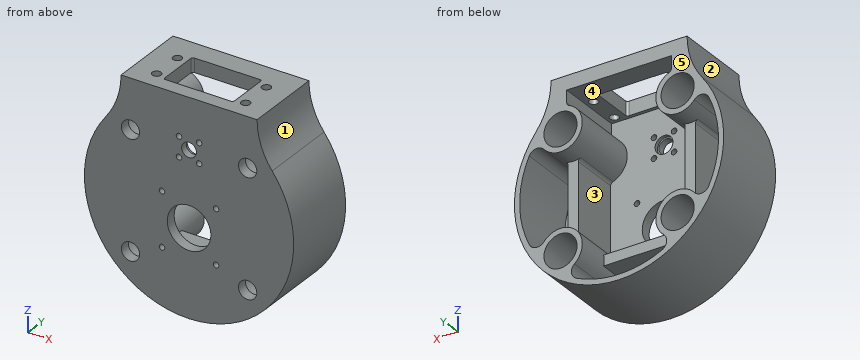
from build123d import *

# Parameters (mm, degrees)
SKETCH1_R           = 9.5
BOSS_EXTRUDE1_DEPTH = 45
BOSS_EXTRUDE2_DEPTH = 6
SKETCH3_R           = 5.25
SKETCH3_R_2         = 4.25
SKETCH3_R_3         = 1.6
CUT_EXTRUDE1_DEPTH  = 95.683683917
FILLET1_R           = 5
SKETCH4_R           = 5.1
CUT_EXTRUDE2_DEPTH  = 2
SKETCH5_R           = 12.5
SKETCH5_R_2         = 1.6
CUT_EXTRUDE3_DEPTH  = 98.308787031
CUT_EXTRUDE4_REACH  = 145.21
SKETCH6_W           = 40
SKETCH6_H           = 25
CUT_EXTRUDE5_REACH  = 145.21
SKETCH7_R           = 2.55
BOSS_EXTRUDE3_DEPTH = 28
FILLET2_R           = 2
BOSS_EXTRUDE4_DEPTH = 20
FILLET3_R           = 1.2


with BuildPart() as part:
    # Sketch1 → Boss-Extrude1 (new body)
    # profile 1 of 3: a face of its own
    with BuildSketch(Plane(origin=(0, 0, 0), x_dir=(1, 0, 0), z_dir=(0, 1, 0))):
        with BuildLine():
            ThreePointArc((-47.647058368, -36.465844689), (-41.21916632, -48.520286728), (-39, -62))
            Line((-39, -62), (39, -62))
            ThreePointArc((39, -62), (41.21916632, -48.520286728), (47.647058368, -36.465844689))
            ThreePointArc((47.647058368, -36.465844689), (0, 60), (-47.647058368, -36.465844689))
        make_face()
        with Locations(Location((-33.587572106, -33.587572106, 0), (0, 0, 90))):
            Circle(SKETCH1_R, mode=Mode.SUBTRACT)
        with Locations(Location((33.587572106, -33.587572106, 0), (0, 0, 90))):
            Circle(SKETCH1_R, mode=Mode.SUBTRACT)
        with BuildLine():
            Line((30, -54), (-30, -54))
            Line((-30, -54), (-30, -48.466483264))
            ThreePointArc((-30, -48.466483264), (-31.792352433, -47.310108082), (-33.540184508, -46.087482283))
            ThreePointArc((-33.540184508, -46.087482283), (-31.751176372, -45.951942317), (-30, -45.561682778))
            ThreePointArc((-30, -45.561682778), (-26.105156211, -23.574408152), (-46.087482283, -33.540184508))
            ThreePointArc((-46.087482283, -33.540184508), (-57, 0), (-46.087482283, 33.540184508))
            ThreePointArc((-46.087482283, 33.540184508), (-24.748737342, 24.748737342), (-33.540184508, 46.087482283))
            ThreePointArc((-33.540184508, 46.087482283), (0, 57), (33.540184508, 46.087482283))
            ThreePointArc((33.540184508, 46.087482283), (24.748737342, 24.748737342), (46.087482283, 33.540184508))
            ThreePointArc((46.087482283, 33.540184508), (57, 0), (46.087482283, -33.540184508))
            ThreePointArc((46.087482283, -33.540184508), (26.105156211, -23.574408152), (30, -45.561682778))
            ThreePointArc((30, -45.561682778), (31.751176372, -45.951942317), (33.540184508, -46.087482283))
            ThreePointArc((33.540184508, -46.087482283), (31.792352433, -47.310108082), (30, -48.466483264))
            Line((30, -48.466483264), (30, -54))
        make_face(mode=Mode.SUBTRACT)
        with Locations(Location((-33.587572106, 33.587572106, 0), (0, 0, 90))):
            Circle(SKETCH1_R, mode=Mode.SUBTRACT)
        with Locations(Location((33.587572106, 33.587572106, 0), (0, 0, 90))):
            Circle(SKETCH1_R, mode=Mode.SUBTRACT)
    # profile 2 of 3: a face of its own
    with BuildSketch(Plane(origin=(0, 0, 0), x_dir=(1, 0, 0), z_dir=(0, 1, 0))):
        with BuildLine():
            Line((30, -45.561682778), (30, -48.466483264))
            ThreePointArc((30, -48.466483264), (31.792352433, -47.310108082), (33.540184508, -46.087482283))
            ThreePointArc((33.540184508, -46.087482283), (31.751176372, -45.951942317), (30, -45.561682778))
        make_face()
    # profile 3 of 3: a face of its own
    with BuildSketch(Plane(origin=(0, 0, 0), x_dir=(1, 0, 0), z_dir=(0, 1, 0))):
        with BuildLine():
            ThreePointArc((-33.540184508, -46.087482283), (-31.792352433, -47.310108082), (-30, -48.466483264))
            Line((-30, -48.466483264), (-30, -45.561682778))
            ThreePointArc((-30, -45.561682778), (-31.751176372, -45.951942317), (-33.540184508, -46.087482283))
        make_face()
    extrude(amount=BOSS_EXTRUDE1_DEPTH)

    # Sketch2 → Boss-Extrude2 (add)
    with BuildSketch(Plane.XZ):
        with BuildLine():
            Line((39, 62), (-39, 62))
            ThreePointArc((-39, 62), (-41.21916632, 48.520286728), (-47.647058368, 36.465844689))
            ThreePointArc((-47.647058368, 36.465844689), (0, -60), (47.647058368, 36.465844689))
            ThreePointArc((47.647058368, 36.465844689), (41.21916632, 48.520286728), (39, 62))
        make_face()
    extrude(amount=-BOSS_EXTRUDE2_DEPTH)

    # Sketch3 → Cut-Extrude1 (cut, through all)
    with BuildSketch(Plane(origin=(0, 6, 0), x_dir=(1, 0, 0), z_dir=(0, 1, 0))):
        with Locations(Location((-33.587572106, 33.587572106, 0), (0, 0, 270))):
            Circle(SKETCH3_R)
        with Locations(Location((33.587572106, 33.587572106, 0), (0, 0, 270))):
            Circle(SKETCH3_R)
        with Locations(Location((33.587572106, -33.587572106, 0), (0, 0, 270))):
            Circle(SKETCH3_R)
        with Locations(Location((-33.587572106, -33.587572106, 0), (0, 0, 270))):
            Circle(SKETCH3_R)
        with Locations(Location((0, -33, 0), (0, 0, 270))):
            Circle(SKETCH3_R_2)
        with Locations(Location((-5.75, -27.25, 0), (0, 0, 270))):
            Circle(SKETCH3_R_3)
        with Locations(Location((5.75, -27.25, 0), (0, 0, 270))):
            Circle(SKETCH3_R_3)
        with Locations(Location((5.75, -38.75, 0), (0, 0, 270))):
            Circle(SKETCH3_R_3)
        with Locations(Location((-5.75, -38.75, 0), (0, 0, 270))):
            Circle(SKETCH3_R_3)
    extrude(amount=-CUT_EXTRUDE1_DEPTH, mode=Mode.SUBTRACT)

    # Fillet1
    fillet1_edges = [part.edges().sort_by_distance(p)[0] for p in [
        (46.087482283, 25.5, 33.540184508),
        (46.087482283, 25.5, -33.540184508),
        (33.540184508, 25.5, -46.087482283),
        (-33.540184508, 25.5, -46.087482283),
        (-46.087482283, 25.5, -33.540184508),
        (-46.087482283, 25.5, 33.540184508),
    ]]
    fillet(fillet1_edges, radius=FILLET1_R)

    # Sketch4 → Cut-Extrude2 (cut)
    with BuildSketch(Plane(origin=(0, 6, 0), x_dir=(1, 0, 0), z_dir=(0, 1, 0))):
        with Locations(Location((0, -33, 0), (0, 0, 270))):
            Circle(SKETCH4_R)
    extrude(amount=-CUT_EXTRUDE2_DEPTH, mode=Mode.SUBTRACT)

    # Sketch5 → Cut-Extrude3 (cut, through all)
    with BuildSketch(Plane.XZ):
        with Locations(Location((0, -10, 0), (0, 0, 270))):
            Circle(SKETCH5_R)
        with Locations(Location((15.5, 5.5, 0), (0, 0, 270))):
            Circle(SKETCH5_R_2)
        with Locations(Location((-15.5, 5.5, 0), (0, 0, 270))):
            Circle(SKETCH5_R_2)
        with Locations(Location((-15.5, -25.5, 0), (0, 0, 270))):
            Circle(SKETCH5_R_2)
        with Locations(Location((15.5, -25.5, 0), (0, 0, 270))):
            Circle(SKETCH5_R_2)
    extrude(amount=-CUT_EXTRUDE3_DEPTH, mode=Mode.SUBTRACT)

    # Sketch6 → Cut-Extrude4 (cut, up to next)
    with BuildSketch(Plane.XY.offset(62), mode=Mode.PRIVATE) as cut_extrude4_sk1:
        with Locations((0, 20.5)):
            Rectangle(SKETCH6_W, SKETCH6_H)
    cut_extrude4_tool1 = extrude(cut_extrude4_sk1.sketch, amount=-CUT_EXTRUDE4_REACH, mode=Mode.PRIVATE) & part.part
    add(cut_extrude4_tool1.solids().sort_by_distance((0, 20.5, 62))[0], mode=Mode.SUBTRACT)

    # Sketch7 → Cut-Extrude5 (cut, up to next)
    with BuildSketch(Plane.XY.offset(62), mode=Mode.PRIVATE) as cut_extrude5_sk1:
        with Locations((-25.5, 10.5)):
            Circle(SKETCH7_R)
    cut_extrude5_tool1 = extrude(cut_extrude5_sk1.sketch, amount=-CUT_EXTRUDE5_REACH, mode=Mode.PRIVATE) & part.part
    # Sketch7 → Cut-Extrude5 (cut, up to next)
    with BuildSketch(Plane.XY.offset(62), mode=Mode.PRIVATE) as cut_extrude5_sk2:
        with Locations((25.5, 10.5)):
            Circle(SKETCH7_R)
    cut_extrude5_tool2 = extrude(cut_extrude5_sk2.sketch, amount=-CUT_EXTRUDE5_REACH, mode=Mode.PRIVATE) & part.part
    # Sketch7 → Cut-Extrude5 (cut, up to next)
    with BuildSketch(Plane.XY.offset(62), mode=Mode.PRIVATE) as cut_extrude5_sk3:
        with Locations((25.5, 28.5)):
            Circle(SKETCH7_R)
    cut_extrude5_tool3 = extrude(cut_extrude5_sk3.sketch, amount=-CUT_EXTRUDE5_REACH, mode=Mode.PRIVATE) & part.part
    # Sketch7 → Cut-Extrude5 (cut, up to next)
    with BuildSketch(Plane.XY.offset(62), mode=Mode.PRIVATE) as cut_extrude5_sk4:
        with Locations((-25.5, 28.5)):
            Circle(SKETCH7_R)
    cut_extrude5_tool4 = extrude(cut_extrude5_sk4.sketch, amount=-CUT_EXTRUDE5_REACH, mode=Mode.PRIVATE) & part.part
    add(cut_extrude5_tool1.solids().sort_by_distance((-25.5, 10.5, 62))[0], mode=Mode.SUBTRACT)
    add(cut_extrude5_tool2.solids().sort_by_distance((25.5, 10.5, 62))[0], mode=Mode.SUBTRACT)
    add(cut_extrude5_tool3.solids().sort_by_distance((25.5, 28.5, 62))[0], mode=Mode.SUBTRACT)
    add(cut_extrude5_tool4.solids().sort_by_distance((-25.5, 28.5, 62))[0], mode=Mode.SUBTRACT)

    # Sketch8 → Boss-Extrude3 (add)
    with BuildSketch(Plane(origin=(0, 6, 0), x_dir=(1, 0, 0), z_dir=(0, 1, 0))):
        with BuildLine():
            Line((-36.587572106, 21.452911007), (-36.587572106, -21.452911007))
            ThreePointArc((-36.587572106, -21.452911007), (-33.587572106, -21.087572106), (-30.587572106, -21.452911007))
            Line((-30.587572106, -21.452911007), (-30.587572106, 21.452911007))
            ThreePointArc((-30.587572106, 21.452911007), (-33.587572106, 21.087572106), (-36.587572106, 21.452911007))
        make_face()
        with BuildLine():
            Line((30.587572106, 21.452911007), (30.587572106, -21.452911007))
            ThreePointArc((30.587572106, -21.452911007), (33.587572106, -21.087572106), (36.587572106, -21.452911007))
            Line((36.587572106, -21.452911007), (36.587572106, 21.452911007))
            ThreePointArc((36.587572106, 21.452911007), (33.587572106, 21.087572106), (30.587572106, 21.452911007))
        make_face()
    extrude(amount=BOSS_EXTRUDE3_DEPTH)

    # Fillet2
    fillet2_edges = [part.edges().sort_by_distance(p)[0] for p in [
        (-30.587572106, 20, -21.452911007),
        (-36.587572106, 20, -21.452911007),
        (-36.587572106, 20, 21.452911007),
        (-30.587572106, 20, 21.452911007),
        (30.587572106, 20, 21.452911007),
        (36.587572106, 20, 21.452911007),
        (36.587572106, 20, -21.452911007),
        (30.587572106, 20, -21.452911007),
        (30, 25.5, 45.561682778),
        (-30, 25.5, 45.561682778),
    ]]
    fillet(fillet2_edges, radius=FILLET2_R)

    # Sketch9 → Boss-Extrude4 (add)
    with BuildSketch(Plane(origin=(0, 6, 0), x_dir=(1, 0, 0), z_dir=(0, 1, 0))):
        with BuildLine():
            Line((-21.452911007, 30.587572106), (21.452911007, 30.587572106))
            ThreePointArc((21.452911007, 30.587572106), (21.087572106, 33.587572106), (21.452911007, 36.587572106))
            Line((21.452911007, 36.587572106), (-21.452911007, 36.587572106))
            ThreePointArc((-21.452911007, 36.587572106), (-21.087572106, 33.587572106), (-21.452911007, 30.587572106))
        make_face()
    extrude(amount=BOSS_EXTRUDE4_DEPTH)

    # Fillet3
    fillet3_edges = [part.edges().sort_by_distance(p)[0] for p in [
        (20, 33, 58),
        (20, 8, 58),
        (-20, 8, 58),
        (-20, 33, 58),
    ]]
    fillet(fillet3_edges, radius=FILLET3_R)


solid = part.part
The listing builds one solid part. Answer for the finished solid, in the listing's coordinates (mm). Face numbers are marked on the shaded views. A direction names the side the tool comes from. Round coordinates to 2 decimals unless told otherwise and drop trailing zeros. Order: outer loops, then holes, each group sorted by start corner. A loop starts at its lowest first (then second) coordinate and runs counter-clockwise, first axis right, second up. Notation, with made-up numbers: M -13.75,58.25 L 3.25,58.25 A24 cw 3.25,76.25 Z; hole C 10,-23 d11. An arc over 180 degrees is marked long. Answer in a Markdown table with one row per item. Add a question column.
1) Consider line 1 along Z through (x, y) = (33, 18); line 2 along X through (y, z) = (29, 9); line 3 along Z through (x, y) = (-34, 11). Determine where each line is inside the solid, lowest interval first. Write a range as from..to.
2) Which of the six approach directions +Z, -Z, +X, -X, +Y, -Y give full straight-line access (tool end or side, diameter ignored) to the marked faces 4 and 5?
3) The part is cut by section C-C on z = -41.5. Determine the outline of the cut face in (x, y), plus the area to 3 significant figures.
4) Flat-ended cylindrical pins translate along their axes: pin 1 Ø19.5 at (x, y) = (-2, 24) entering from -Z; pin 2 Ø3 at (x, z) = (5.75, 27.25) entering from +Y; pin 3 Ø1.5 at (y, z) = (11.5, -19.5) entering from -X; pin 4 Ø8 at (x, y) = (45.5, 26.5) entering from -Z. Find the tip coordinate at first contact, or state that the pin passes through.
5) Determine the mould class of the marked faces 1, 2 and 3 for opening direction X: pulls with the +X half, pulls with the -X half, needs draft (parallel to the pull), parting line crosses it, or undercut.
6) The part is cut by section D-D on y = 16.5. Count the separate pieces of the cut face and the enclosed holes in it, plus the area to 3 significant figures.
7) The part is cut by section B-B on z = 0. Determine the outline of the cut face in (x, y).
8) The part is cut by section A-A on x = 0. Determine the outline of the cut face in (y, z).
Findings below:
| question | item | result |
|---|---|---|
| 1 | line 1 | z = -50.11..-43.07, -24.11..24.11, 43.07..62 |
| 1 | line 2 | x = -59.32..-56.28, -36.59..-30.59, 30.59..36.59, 56.28..59.32 |
| 1 | line 3 | z = -49.44..-43.08, -24.1..24.1, 43.08..62 |
| 2 | face 4 | +Y |
| 2 | face 5 | +Z, -Z, +X, -X, +Y |
| 3 | outline | M -43.33,0 L 43.33,0 L 43.33,45 L 38.85,45 L 38.85,6 L 28.33,6 L 28.33,45 L 23.91,45 L 23.91,6 L -23.91,6 L -23.91,45 L -28.33,45 L -28.33,6 L -38.85,6 L -38.85,45 L -43.33,45 Z |
| 3 | area | 1,210 mm² |
| 4 | pin 1 | stops at z = -60 |
| 4 | pin 2 | passes through |
| 4 | pin 3 | stops at x = -57 |
| 4 | pin 4 | stops at z = -43.33 |
| 5 | face 1 | pulls with the +X half |
| 5 | face 2 | pulls with the -X half |
| 5 | face 3 | undercut |
| 6 | separate pieces | 1 |
| 6 | enclosed holes | 7 |
| 6 | area | 2,940 mm² |
| 7 | outline | M -60,0 L -7.5,0 L -7.5,6 L -30.59,6 L -30.59,34 L -36.59,34 L -36.59,6 L -57,6 L -57,45 L -60,45 Z; M 7.5,0 L 60,0 L 60,45 L 57,45 L 57,6 L 36.59,6 L 36.59,34 L 30.59,34 L 30.59,6 L 7.5,6 Z |
| 8 | outline | M 0,-60 L 45,-60 L 45,-57 L 6,-57 L 6,-36.59 L 26,-36.59 L 26,-30.59 L 6,-30.59 L 6,-22.5 L 0,-22.5 Z; M 0,2.5 L 6,2.5 L 6,27.9 L 4,27.9 L 4,28.75 L 0,28.75 Z; M 0,37.25 L 4,37.25 L 4,38.1 L 6,38.1 L 6,54 L 8,54 L 8,62 L 0,62 Z; M 33,54 L 45,54 L 45,62 L 33,62 Z |
